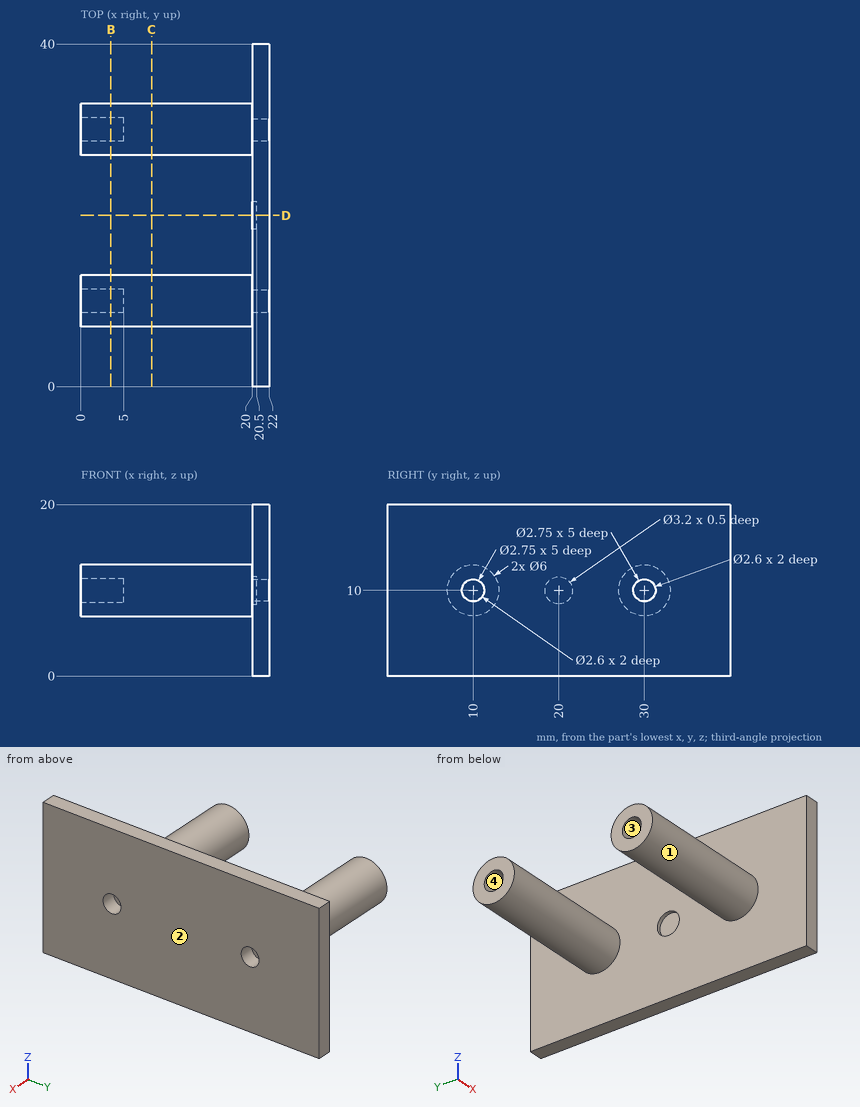
For this review, use the dimensioned drawing (mm, ordinates from the lowest corner) and the shaded views. Round coordinates to 2 decimals unless told otherwise and drop trailing zeros. Write each loop counter-clockwise with the first axis right and the second up, starting at its lowest first coordinate (ties: lowest second). Pieces come first, ordered by that corner, then holes. Notation, with made-up numbers: (73, 28) -> (88, 28) arc R26 cw to (88, 62) -> close; hole circle Ø5 at (-6, 65.25). An arc over 180 degrees is marked (long way). One line per item, written item: value. Start each with the question number.
Q1. The part is to be moulded in two halves that separate along Z. For the marked faces 1, 2, 3 and 4, say which applies: pulls with the +Z half, pulls with the -Z half, needs draft (parallel to the pull), parting line crosses it, or undercut.
Q2. To check wall thickness, follow probe 1 along Y at (x, z) = (2.8, 10) (3 decimals); probe 2 along Y at (x, z) = (21.2, 10); probe 3 along Z at (x, y) = (2.85, 10) (3 decimals). State the ranges of each line that lie inside material, in increasing order.
Q3. Add section C-C (x = 8.25). Give the boundary of the cut face in (y, z).
Q4. Add section D-D (y = 20). Give the boundary of the cut face in (x, z).
Q5. Add section B-B (x = 3.5). Give the boundary of the cut face in (y, z) (3 decimals).
Q6. Insertion check: P1, Ø6, axis at x = 16, y = 23.5, coming from the -Z side (3 decimals); P2, Ø3.5, axis at y = 20, z = 10.5, coming from the -X side; P3, Ø3, axis at x = 18, z = 13, coming from the +Y side; P4, Ø10, axis at x = 4.5, z = 7.5, coming from the -Y side. Each pin has a flat end and moves straight along its axis. Give the tip position at first contact, or say it passes through.
Response:
1. face 1: parting line crosses it
1. face 2: needs draft
1. face 3: undercut
1. face 4: undercut
2. probe 1: y = 7 to 8.625, 11.375 to 13, 27 to 28.625, 31.375 to 33
2. probe 2: y = 0 to 8.7, 11.3 to 28.7, 31.3 to 40
2. probe 3: z = 7 to 8.625, 11.375 to 13
3. outline: circle Ø6 at (10, 10); circle Ø6 at (30, 10)
4. outline: (20, 0) -> (22, 0) -> (22, 20) -> (20, 20) -> (20, 11.6) -> (20.5, 11.6) -> (20.5, 8.4) -> (20, 8.4) -> close
5. outline: circle Ø6 at (10, 10); circle Ø6 at (30, 10); hole circle Ø2.75 at (10, 10); hole circle Ø2.75 at (30, 10)
6. P1: passes through
6. P2: stops at x = 20
6. P3: stops at y = 32.6
6. P4: stops at y = 7
